Design review of the part built by this model. Coordinates are the model's own, in mm. Face numbers are marked on the shaded views. Round coordinates to 2 decimals unless told otherwise and drop trailing zeros. Order: outer loops, then holes, each group sorted by start corner. A loop starts at its lowest first (then second) coordinate and runs counter-clockwise, first axis right, second up. Notation, with made-up numbers: (39.5, 11) - (75.5, 11) arc R15 cw to (75.5, 15) - close; hole circle Ø2 at (22, 25). An arc over 180 degrees is marked (long way). Write item = value, one per line.
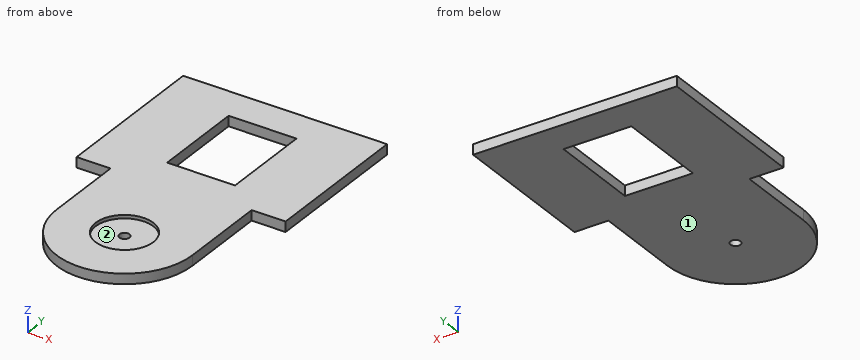
from build123d import *

# Parameters (mm, degrees)
CROQUIS1_R              = 1.5
CROQUIS1_W              = 20
CROQUIS1_H              = 27.278528679
SALIENTE_EXTRUIR1_DEPTH = 3
CROQUIS2_R              = 8.5
CORTAR_EXTRUIR1_DEPTH   = 1


with BuildPart() as part:
    # Croquis1 → Saliente-Extruir1 (new body)
    with BuildSketch(Plane.XY):
        with BuildLine():
            Line((-113.991811363, 10.970788205), (-113.991811363, 34.958108792))
            Line((-113.991811363, 34.958108792), (-123.991811363, 34.958108792))
            Line((-123.991811363, 34.958108792), (-123.991811363, 82.236637471))
            Line((-123.991811363, 82.236637471), (-63.991811363, 82.236637471))
            Line((-63.991811363, 82.236637471), (-63.991811363, 37.236637471))
            Line((-63.991811363, 37.236637471), (-73.991811363, 37.236637471))
            Line((-73.991811363, 37.236637471), (-73.991811363, 10.970788205))
            ThreePointArc((-73.991811363, 10.970788205), (-93.991811363, -9.029211795), (-113.991811363, 10.970788205))
        make_face()
        with Locations((-93.991811363, 10.970788205)):
            Circle(CROQUIS1_R, mode=Mode.SUBTRACT)
        with Locations((-93.991811363, 58.597373132)):
            Rectangle(CROQUIS1_W, CROQUIS1_H, mode=Mode.SUBTRACT)
    extrude(amount=SALIENTE_EXTRUIR1_DEPTH)

    # Croquis2 → Cortar-Extruir1 (cut)
    with BuildSketch(Plane.XY.offset(3)):
        with Locations((-93.991811363, 10.970788205)):
            Circle(CROQUIS2_R)
    extrude(amount=-CORTAR_EXTRUIR1_DEPTH, mode=Mode.SUBTRACT)


solid = part.part
1) We need section B-B on z = 2.5. Write out the cut boundary in (x, y).
Findings:
outline = (-123.99, 34.96) - (-113.99, 34.96) - (-113.99, 10.97) arc R20 ccw to (-73.99, 10.97) - (-73.99, 37.24) - (-63.99, 37.24) - (-63.99, 82.24) - (-123.99, 82.24) - close; hole (-103.99, 44.96) - (-83.99, 44.96) - (-83.99, 72.24) - (-103.99, 72.24) - close; hole circle Ø17 at (-93.99, 10.97)
2) To check wall thickness, follow L1, parallel to X at y = 61, z = 1.1; L2, parallel to X at y = 11, z = 1.4; L3, parallel to Y at x = -116.5, z = 2.5. State the ranges of each line that lie inside material, in increasing order. Write a range as from..to.
Findings:
L1 = -123.99..-103.99, -83.99..-63.99
L2 = -113.99..-95.49, -92.49..-73.99
L3 = 34.96..82.24
3) We need section D-D on x = -88.5. Write out the cut boundary in (y, z), and give its area (3 significant figures).
Findings:
outline = (-8.26, 0) - (44.96, 0) - (44.96, 3) - (17.46, 3) - (17.46, 2) - (4.48, 2) - (4.48, 3) - (-8.26, 3) - close; (72.24, 0) - (82.24, 0) - (82.24, 3) - (72.24, 3) - close
area = 177 mm^2
4) We need section A-A on y = 55. Write out the cut boundary in (x, z).
Findings:
outline = (-123.99, 0) - (-103.99, 0) - (-103.99, 3) - (-123.99, 3) - close; (-83.99, 0) - (-63.99, 0) - (-63.99, 3) - (-83.99, 3) - close
5) We need section C-C on x = -97. Write out the cut boundary in (y, z).
Findings:
outline = (-8.8, 0) - (44.96, 0) - (44.96, 3) - (18.92, 3) - (18.92, 2) - (3.02, 2) - (3.02, 3) - (-8.8, 3) - close; (72.24, 0) - (82.24, 0) - (82.24, 3) - (72.24, 3) - close
6) The part is to be moulded in two halves that separate along Y. For the marked faces 1 and 2, say which applies: released by +Y, released by -Y, zero draft, split by the parting line, or undercut.
Findings:
face_1 = zero draft
face_2 = undercut
7) Clearance check with flat-ended pins moving along their axes: pin 1 Ø1.5 at (y, z) = (24, 1) entering from +X; pin 2 Ø5 at (x, y) = (-98, 7.5) entering from +Z; pin 3 Ø1.8 at (x, y) = (-93.99, 10.97) entering from +Z; pin 4 Ø1.5 at (x, z) = (-119, 2) entering from -Y. State where each tip first meets the part, or that it passes through.
Findings:
pin_1 = -73.99
pin_2 = 2
pin_3 = through
pin_4 = 34.96
